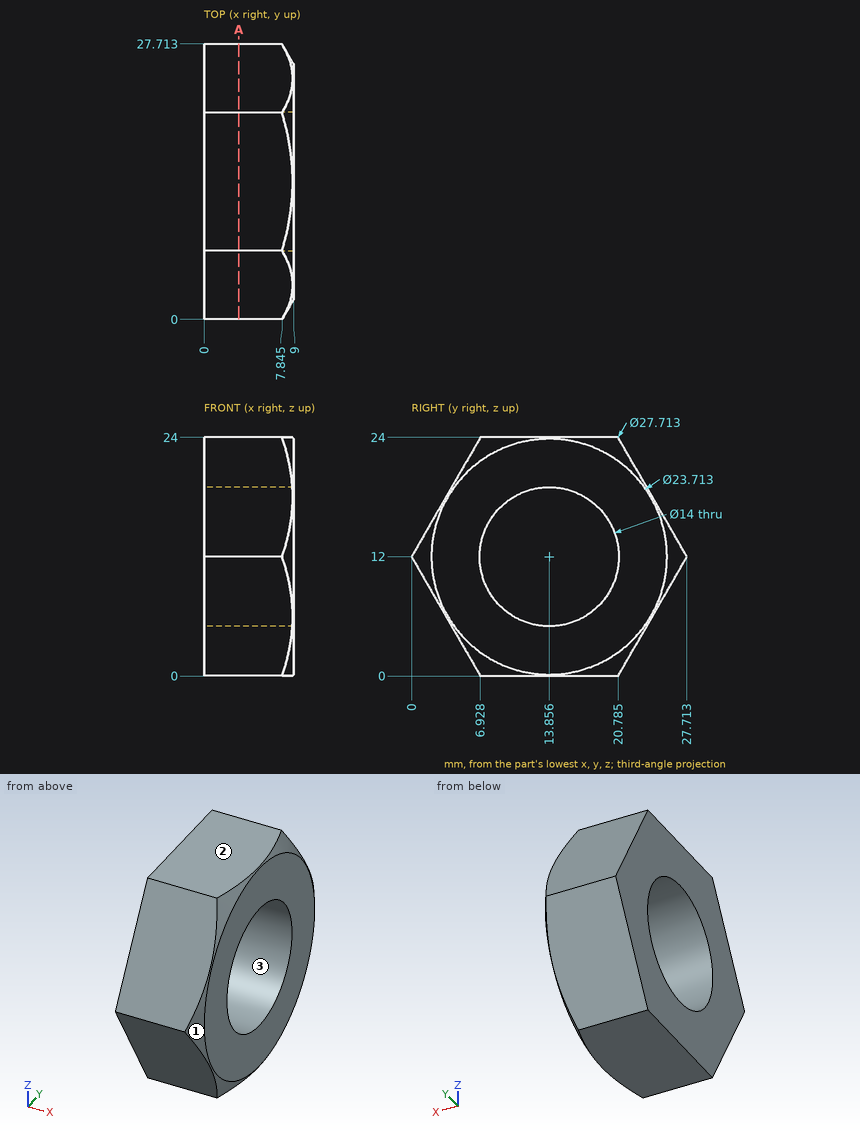
Design review of the part shown in the three views and the two pictorial views. Dimensions are in mm from the part's minimum x, y and z. Give positions to 0.01 mm unless a question says otherwise; leave off trailing zeros. Loops run counter-clockwise (first coordinate to the right, second up) from the corner with the lowest first, then second, coordinate; pieces in that order, holes last. Notation, with made-up numbers: (26.5, 49.5) -> (62.5, 49.5) arc R30 ccw to (62.5, 71.5) -> close; hole circle Ø11 at (85.5, 35). An arc over 180 degrees is marked (long way). Put each result on its own line as item: value. Start each with the question number.
1. Mouldability with a two-part tool opening along Y and no side actions: class the marked faces 1, 2 and 3 as released by +Y, released by -Y, zero draft, split by the parting line, or undercut.
2. Wall thickness on probe 1 along Y at (x, z) = (2.75, 13.25) (1 decimal); probe 2 along Y at (x, z) = (7.25, 9.75) (1 decimal); probe 3 along Z at (x, y) = (8.75, 19.5) (1 decimal): over which ranges is each line inside the solid? List them lowest first.
3. We need section A-A on x = 3.5. State the section outline as (y, z) points (1 decimal), then the cut area to 3 significant figures.
4. Clearance check with flat-ended pins moving along their axes: P1, Ø4, axis at x = 3, z = 18, coming from the +Y side; P2, Ø1.5, axis at x = 2.5, z = 7, coming from the +Y side; P3, Ø1.5, axis at x = 6, z = 4, coming from the -Y side (1 decimal); P4, Ø8.5, axis at y = 13.86, z = 12, coming from the +X side. State where each tip first meets the part, or that it passes through.
Determined:
1. face 1: split by the parting line
1. face 2: zero draft
1. face 3: undercut
2. probe 1: 0.7 to 7, 20.7 to 27
2. probe 2: 1.3 to 7.2, 20.5 to 26.4
2. probe 3: 1.1 to 7.9, 16.1 to 22.9
3. outline: (0, 12) -> (6.9, 0) -> (20.8, 0) -> (27.7, 12) -> (20.8, 24) -> (6.9, 24) -> close; hole circle Ø14 at (13.9, 12)
3. area: 345 mm^2
4. P1: y = 25.4
4. P2: y = 25.26
4. P3: y = 4.2
4. P4: through
